Build history of the part. All positions in model axes, mm. Face numbers are marked on the shaded views. Coordinates: 2 decimals unless noted, no trailing zeros. Order: outer loops, then holes, each group sorted by start corner. A loop starts at its lowest first (then second) coordinate and runs counter-clockwise, first axis right, second up. Notation, with made-up numbers: (-40, 26) - (4, 26) arc R18 cw to (4, 34) - close; hole circle Ø4 at (8, 38.25). An arc over 180 degrees is marked (long way). One line per item, written item: value.
from build123d import *

# Parameters (mm, degrees)
SKETCH1_R           = 1
SKETCH1_R_2         = 1.5
BOSS_EXTRUDE1_DEPTH = 2
SKETCH2_R           = 4
SKETCH2_R_2         = 2.5
BOSS_EXTRUDE2_DEPTH = 5
BOSS_EXTRUDE3_START = 1
SKETCH3_R           = 6
SKETCH3_R_2         = 4
BOSS_EXTRUDE3_DEPTH = 1
SKETCH4_R           = 3.5
CUT_EXTRUDE1_DEPTH  = 1
SKETCH5_W           = 12
SKETCH5_H           = 1
BOSS_EXTRUDE4_DEPTH = 1
CUT_EXTRUDE2_DEPTH  = 20


with BuildPart() as part:
    # Sketch1 → Boss-Extrude1 (new body)
    # profile 1 of 3: a face of its own
    with BuildSketch(Plane(origin=(0, 0, 0), x_dir=(1, 0, 0), z_dir=(0, 1, 0))):
        with BuildLine():
            Line((-1.075862069, 6.410344828), (-24, 4.5))
            ThreePointArc((-24, 4.5), (-28.5, 0), (-24, -4.5))
            Line((-24, -4.5), (-1.075862069, -6.410344828))
            ThreePointArc((-1.075862069, -6.410344828), (-6.5, 0), (-1.075862069, 6.410344828))
        make_face()
        with Locations(Location((-21, 0, 0), (0, 0, 270))):
            Circle(SKETCH1_R, mode=Mode.SUBTRACT)
        with Locations(Location((-18, 0, 0), (0, 0, 270))):
            Circle(SKETCH1_R, mode=Mode.SUBTRACT)
        with Locations(Location((-15, 0, 0), (0, 0, 270))):
            Circle(SKETCH1_R, mode=Mode.SUBTRACT)
        with Locations(Location((-12, 0, 0), (0, 0, 270))):
            Circle(SKETCH1_R, mode=Mode.SUBTRACT)
        with Locations(Location((-9, 0, 0), (0, 0, 270))):
            Circle(SKETCH1_R, mode=Mode.SUBTRACT)
        with Locations(Location((-24, 0, 0), (0, 0, 270))):
            Circle(SKETCH1_R, mode=Mode.SUBTRACT)
    # profile 2 of 3: a face of its own
    with BuildSketch(Plane(origin=(0, 0, 0), x_dir=(1, 0, 0), z_dir=(0, 1, 0))):
        with BuildLine():
            Line((0, 6.5), (-1.075862069, 6.410344828))
            ThreePointArc((-1.075862069, 6.410344828), (-6.5, 0), (-1.075862069, -6.410344828))
            Line((-1.075862069, -6.410344828), (0, -6.5))
            Line((0, -6.5), (1.075862069, -6.410344828))
            ThreePointArc((1.075862069, -6.410344828), (4.962010855, -4.19862457), (6.5, 0))
            ThreePointArc((6.5, 0), (4.962010855, 4.19862457), (1.075862069, 6.410344828))
            Line((1.075862069, 6.410344828), (0, 6.5))
        make_face()
        with Locations(Location((0, 0, 0), (0, 0, 270))):
            Circle(SKETCH1_R_2, mode=Mode.SUBTRACT)
    # profile 3 of 3: a face of its own
    with BuildSketch(Plane(origin=(0, 0, 0), x_dir=(1, 0, 0), z_dir=(0, 1, 0))):
        with BuildLine():
            Line((24, 4.5), (1.075862069, 6.410344828))
            ThreePointArc((1.075862069, 6.410344828), (4.962010855, 4.19862457), (6.5, 0))
            ThreePointArc((6.5, 0), (4.962010855, -4.19862457), (1.075862069, -6.410344828))
            Line((1.075862069, -6.410344828), (24, -4.5))
            ThreePointArc((24, -4.5), (28.5, 0), (24, 4.5))
        make_face()
        with Locations(Location((9, 0, 0), (0, 0, 270))):
            Circle(SKETCH1_R, mode=Mode.SUBTRACT)
        with Locations(Location((12, 0, 0), (0, 0, 270))):
            Circle(SKETCH1_R, mode=Mode.SUBTRACT)
        with Locations(Location((15, 0, 0), (0, 0, 270))):
            Circle(SKETCH1_R, mode=Mode.SUBTRACT)
        with Locations(Location((18, 0, 0), (0, 0, 270))):
            Circle(SKETCH1_R, mode=Mode.SUBTRACT)
        with Locations(Location((21, 0, 0), (0, 0, 270))):
            Circle(SKETCH1_R, mode=Mode.SUBTRACT)
        with Locations(Location((24, 0, 0), (0, 0, 270))):
            Circle(SKETCH1_R, mode=Mode.SUBTRACT)
    extrude(amount=BOSS_EXTRUDE1_DEPTH)

    # Sketch2 → Boss-Extrude2 (add)
    with BuildSketch(Plane(origin=(0, 2, 0), x_dir=(1, 0, 0), z_dir=(0, 1, 0))):
        with Locations(Location((0, 0, 0), (0, 0, 270))):
            Circle(SKETCH2_R)
        with Locations(Location((0, 0, 0), (0, 0, 270))):
            Circle(SKETCH2_R_2, mode=Mode.SUBTRACT)
    extrude(amount=BOSS_EXTRUDE2_DEPTH)

    # Sketch3 → Boss-Extrude3 (add)
    with BuildSketch(Plane.XZ.offset(BOSS_EXTRUDE3_START)):
        with Locations(Location((0, 0, 0), (0, 0, 90))):
            Circle(SKETCH3_R)
        with Locations(Location((0, 0, 0), (0, 0, 90))):
            Circle(SKETCH3_R_2, mode=Mode.SUBTRACT)
    extrude(amount=-BOSS_EXTRUDE3_DEPTH)

    # Sketch4 → Cut-Extrude1 (cut)
    with BuildSketch(Plane.XZ):
        with Locations(Location((0, 0, 0), (0, 0, 270))):
            Circle(SKETCH4_R)
    extrude(amount=-CUT_EXTRUDE1_DEPTH, mode=Mode.SUBTRACT)

    # Sketch5 → Boss-Extrude4 (add)
    with BuildSketch(Plane(origin=(0, 2, 0), x_dir=(1, 0, 0), z_dir=(0, 1, 0))):
        with Locations((0, 5.5)):
            Rectangle(SKETCH5_W, SKETCH5_H)
        with Locations((0, -5.5)):
            Rectangle(SKETCH5_W, SKETCH5_H)
    extrude(amount=BOSS_EXTRUDE4_DEPTH)

    # Sketch6 → Cut-Extrude2 (cut)
    with BuildSketch(Plane.XY.offset(6)):
        Polygon((-4, 3), (-6, 2), (-6, 3), align=None)
        Polygon((6, 2), (4, 3), (6, 3), align=None)
    extrude(amount=-CUT_EXTRUDE2_DEPTH, mode=Mode.SUBTRACT)


solid = part.part
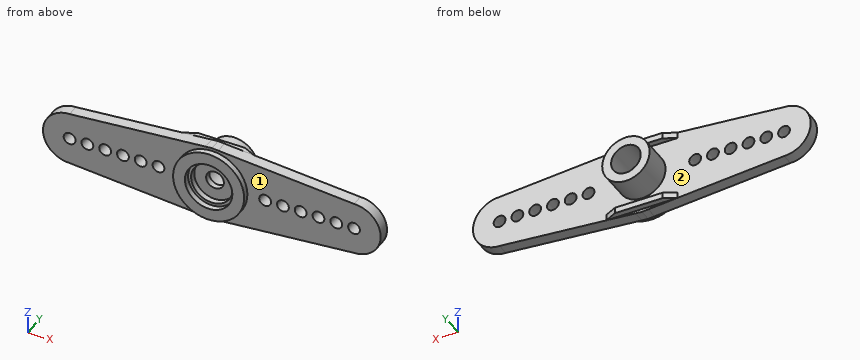
1. Band-saw the part on C-C, the plane y = 6. Give the cut face in (x, z), and give its area (3 significant figures).
Values found:
outline: circle Ø8 at (0, 0); hole circle Ø5 at (0, 0)
area: 30.6 mm2
2. Band-saw the part on D-D, the plane z = 0. Count the separate pieces of the cut face and the enclosed holes in it, and give its area (3 significant figures).
Values found:
separate pieces: 14
enclosed holes: 0
area: 75.0 mm2
3. Band-saw the part on B-B, the plane x = 21. Give the cut face in (y, z), and give its area (3 significant figures).
Values found:
outline: (0, -4.75) - (2, -4.75) - (2, -1) - (0, -1) - close; (0, 1) - (2, 1) - (2, 4.75) - (0, 4.75) - close
area: 15.0 mm2
4. Two-plate mould, pull along Z, no slides. Class the marked faces 1 and 2: pulls with the +Z half, pulls with the -Z half, needs draft (parallel to the pull), parting line crosses it, or undercut.
Values found:
face 1: needs draft
face 2: undercut
5. Band-saw the part on A-A, the plane x = 15. Give the cut face in (y, z).
Values found:
outline: (0, -5.25) - (2, -5.25) - (2, -1) - (0, -1) - close; (0, 1) - (2, 1) - (2, 5.25) - (0, 5.25) - close
6. Probe line 1 along Z through (x, y) = (0, 1.4); line 2 along Y through (x, z) = (-3.5, 3); line 3 along Y through (x, z) = (16, 1.5). List the from-to ranges inside material, lowest first.
Values found:
line 1: z = -6.5 to -1.5, 1.5 to 6.5
line 2: y = -1 to 2
line 3: y = 0 to 2
7. Flat gauge pins, fed straight in: P1, Ø1.6, axis at x = 9, z = 0, coming from the +Y side; P2, Ø3, axis at x = -18, z = 0, coming from the +Y side; P3, Ø2, axis at x = 10.5, z = -2.5, coming from the -Y side; P4, Ø0.5, axis at x = -2, y = 2.5, coming from the +Z side. Where does each tip first touch, or does it go through?
Values found:
P1: passes through
P2: stops at y = 2
P3: stops at y = 0
P4: stops at z = 6
